```python
from build123d import *

# Parameters (mm, degrees)
F0_W     = 50.8
F0_H     = 6.35
F1_DEPTH = 152.4
F0_R     = 3.175
F2_DEPTH = 6.35
F3_R     = 10.16
F4_R     = 10.16


with BuildPart() as f1:
    # F0 (on Front) → F1 (new body)
    with BuildSketch(Plane.XZ):
        with Locations((0, 33.433512)):
            Rectangle(F0_W, F0_H)
    extrude(amount=F1_DEPTH)

    # F0 (on Front) → F2 (join)
    with BuildSketch(Plane.XZ):
        Polygon((-12.7, 284.258512), (-25.4, 262.963444), (-25.4, 36.608512), (25.4, 36.608512), (25.4, 262.963444), (12.7, 284.258512), (0, 284.258512), align=None)
        with Locations((18.223565, 73.40546)):
            Circle(F0_R, mode=Mode.SUBTRACT)
        with Locations((-18.311808, 173.985869)):
            Circle(F0_R, mode=Mode.SUBTRACT)
        with BuildLine():
            ThreePointArc((6.35, 252.508512), (-4.490128, 248.018384), (0, 258.858512))
            ThreePointArc((0, 258.858512), (4.490128, 256.99864), (6.35, 252.508512))
        make_face(mode=Mode.SUBTRACT)
    extrude(amount=F2_DEPTH)

    # F3
    f3_edges = [f1.edges().sort_by_distance(p)[0] for p in [
        (0, -6.35, 36.608512),
        (0, 0, 30.258512),
    ]]
    fillet(f3_edges, radius=F3_R)

    # F4
    f4_edges = [f1.edges().sort_by_distance(p)[0] for p in [
        (-25.4, -152.4, 33.433512),
        (25.4, -152.4, 33.433512),
    ]]
    fillet(f4_edges, radius=F4_R)


solid = f1.part
```
Input: part model. Units: mm. Frame: model coordinates. Coordinates: 2 decimals unless noted, no trailing zeros. Loops run counter-clockwise (first coordinate to the right, second up) from the corner with the lowest first, then second, coordinate; pieces in that order, holes last. Notation, with made-up numbers: (-4, 85.25) - (38, 85.25) arc R18 cw to (38, 100.25) - close; hole circle Ø3 at (23.25, 76). An arc over 180 degrees is marked (long way). Answer in a Markdown table with one row per item.
(1) Pin query (flat end, axial travel): P1, Ø5, axis at x = -14.5, y = -100.5, coming from the +Z side; P2, Ø1, axis at x = 15, z = 74, coming from the -Y side; P3, Ø5.5, axis at x = 18.22, z = 73.41, coming from the +Y side. Return the tip coordinate at first contact, or that it passes through.
Model answer:
| item | result |
|---|---|
| P1 | stops at z = 36.61 |
| P2 | stops at y = -6.35 |
| P3 | passes through |
(2) Cut plane A-A on z = 117. Output: boundary loops of the cut face in (x, y).
Model answer:
| item | result |
|---|---|
| outline | (-25.4, -6.35) - (25.4, -6.35) - (25.4, 0) - (-25.4, 0) - close |
(3) Cut plane B-B on y = -114. Output: boundary loops of the cut face in (x, z).
Model answer:
| item | result |
|---|---|
| outline | (-25.4, 30.26) - (25.4, 30.26) - (25.4, 36.61) - (-25.4, 36.61) - close |
(4) Material intervals for L1, parallel to Y at x = -1.5, z = 141; L2, parallel to Z at x = 3.5, y = -63, sorted ascending. Write a range as from..to.
Model answer:
| item | result |
|---|---|
| L1 | y = -6.35..0 |
| L2 | z = 30.26..36.61 |
(5) Mould query, pull axis Z, two halves, no side actions, for faces 1 (the face through (0, -80, 30.259)), 2 (the face through (17.81, -3.131, 76.553)), 3 (the face through (0, -84, 36.609)), 4 (the face through (0, -6.35, 167)). Classes: pulls with the +Z half, pulls with the -Z half, needs draft (parallel to the pull), parting line crosses it, or undercut.
Model answer:
| item | result |
|---|---|
| face 1 | pulls with the -Z half |
| face 2 | undercut |
| face 3 | pulls with the +Z half |
| face 4 | needs draft |
